```python
from build123d import *

# Parameters (mm, degrees)
EXTRUDE_1_DEPTH        = 330
SKETCH_2_R             = 3
SKETCH_2_R_2           = 1.75
CUT_EXTRUDE_1_DEPTH    = 4.5
SKETCH_2_2_R           = 1.75
CUT_EXTRUDE_2_DEPTH    = 9
PATTERN_LINEAR_1_COUNT = 16
PATTERN_LINEAR_1_PITCH = 25


with BuildPart() as part:
    # Эскиз1 → Бобышка-Вытянуть1 (new body)
    with BuildSketch(Plane.XY):
        with BuildLine():
            Line((-6, 3.7), (-5.7, 4))
            Line((-5.7, 4), (5.7, 4))
            Line((5.7, 4), (6, 3.7))
            Line((6, 3.7), (6, 2.451013544))
            ThreePointArc((6, 2.451013544), (5.597935912, 2.202976267), (5.354599002, 1.798050138))
            Line((5.354599002, 1.798050138), (4.643514056, 1.798050138))
            Line((4.643514056, 1.798050138), (4.643514056, 1.201949862))
            Line((4.643514056, 1.201949862), (5.354599002, 1.201949862))
            ThreePointArc((5.354599002, 1.201949862), (5.597935912, 0.797023733), (6, 0.548986456))
            Line((6, 0.548986456), (6, -3.7))
            Line((6, -3.7), (5.7, -4))
            Line((5.7, -4), (-5.7, -4))
            Line((-5.7, -4), (-6, -3.7))
            Line((-6, -3.7), (-6, 0.548986456))
            ThreePointArc((-6, 0.548986456), (-5.597935912, 0.797023733), (-5.354599002, 1.201949862))
            Line((-5.354599002, 1.201949862), (-4.643514056, 1.201949862))
            Line((-4.643514056, 1.201949862), (-4.643514056, 1.798050138))
            Line((-4.643514056, 1.798050138), (-5.354599002, 1.798050138))
            ThreePointArc((-5.354599002, 1.798050138), (-5.597935912, 2.202976267), (-6, 2.451013544))
            Line((-6, 2.451013544), (-6, 3.7))
        make_face()
    extrude(amount=EXTRUDE_1_DEPTH)

    # Эскиз2 → Вырез-Вытянуть1 (cut)
    with BuildSketch(Plane(origin=(0, 4, 0), x_dir=(1, 0, 0), z_dir=(0, 1, 0))):
        with Locations((0, -12)):
            Circle(SKETCH_2_R)
        with Locations((0, -12)):
            Circle(SKETCH_2_R_2, mode=Mode.SUBTRACT)
    cut_extrude_1 = extrude(amount=-CUT_EXTRUDE_1_DEPTH, mode=Mode.SUBTRACT)

    # Эскиз2<2> → Вырез-Вытянуть2 (cut, through all)
    with BuildSketch(Plane(origin=(0, 4, 0), x_dir=(1, 0, 0), z_dir=(0, 1, 0))):
        with Locations((0, -12)):
            Circle(SKETCH_2_2_R)
    cut_extrude_2 = extrude(amount=-CUT_EXTRUDE_2_DEPTH, mode=Mode.SUBTRACT)

    # Линейный массив1: Вырез-Вытянуть1, Вырез-Вытянуть2 ×16
    with Locations(*[(0, 0, i * PATTERN_LINEAR_1_PITCH) for i in range(1, PATTERN_LINEAR_1_COUNT)]):
        add(cut_extrude_1, mode=Mode.SUBTRACT)
        add(cut_extrude_2, mode=Mode.SUBTRACT)


solid = part.part
```
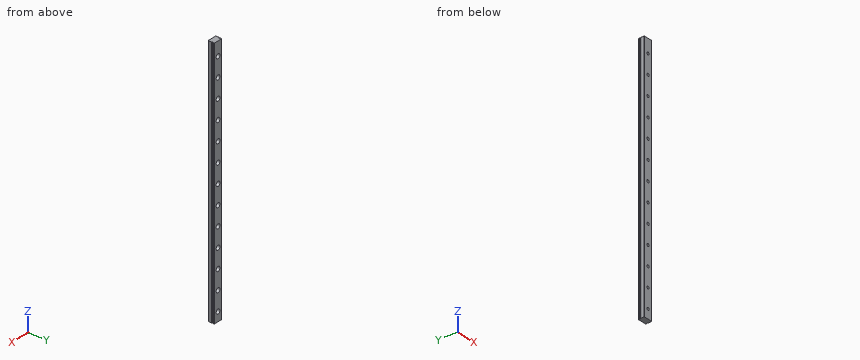
Can you work these out from the model? Positions are in its coordinate system, mm. Give positions to 0.01 mm unless a question says otherwise; leave off trailing zeros. Loops run counter-clockwise (first coordinate to the right, second up) from the corner with the lowest first, then second, coordinate; pieces in that order, holes last. Notation, with made-up numbers: M 19,-14 L 58,-14 A28 ccw 58,5 Z; hole C 2,-25.75 d6. An arc over 180 degrees is marked long. Answer in a Markdown table with one row per item.
1. Suppose I cut it at A-A on z = 253.5. Write out the boundary of the cut face in (x, y), plus the area to 3 significant figures.
Taken from the geometry:
| item | result |
|---|---|
| outline | M -6,-3.7 L -5.7,-4 L 5.7,-4 L 6,-3.7 L 6,0.55 A1 cw 5.35,1.2 L 4.64,1.2 L 4.64,1.8 L 5.35,1.8 A1 cw 6,2.45 L 6,3.7 L 5.7,4 L -5.7,4 L -6,3.7 L -6,2.45 A1 cw -5.35,1.8 L -4.64,1.8 L -4.64,1.2 L -5.35,1.2 A1 cw -6,0.55 Z |
| area | 93.1 mm² |
2. If I drill on line 1 along Y through (x, z) = (5, 292); line 2 along X through (y, z) = (0.5, 287); line 3 along Y through (x, z) = (0.75, 264.5), over which ranges is the centre line in solid material (lowest first)?
Taken from the geometry:
| item | result |
|---|---|
| line 1 | y = -4 to 1.2, 1.8 to 4 |
| line 2 | x = -6 to -3, 3 to 6 |
| line 3 | y = -4 to -0.5 |
3. For pin 1 Ø1.8 at (x, z) = (1, 211) entering from +Y; pin 2 Ø0.5 at (y, z) = (1.5, 181) entering from -X, each with a flat end and sliding along its axis, tell me the tip position at first contact or that it passes through.
Taken from the geometry:
| item | result |
|---|---|
| pin 1 | stops at y = -0.5 |
| pin 2 | stops at x = -4.64 |
